Can you work these out from the model? Positions are in its coordinate system, mm. Give positions to 0.01 mm unless a question says otherwise; leave off trailing zeros. Loops run counter-clockwise (first coordinate to the right, second up) from the corner with the lowest first, then second, coordinate; pieces in that order, holes last. Notation, with made-up numbers: M -12.5,60 L 7.5,60 A24 ccw 7.5,76 Z; hole C 82,65 d4. An arc over 180 degrees is marked long. One line per item, written item: value. Start each with the question number.
from build123d import *

# Parameters (mm, degrees)
F0_W     = 5
F0_H     = 5
F1_DEPTH = 65
F2_SIZE  = 1
F3_R     = 0.65
F4_DEPTH = 6


with BuildPart() as f1:
    # F0 (on Top) → F1 (new body)
    with BuildSketch(Plane.XY):
        Rectangle(F0_W, F0_H)
    extrude(amount=F1_DEPTH)

    # F2
    f2_edges = [f1.edges().sort_by_distance(p)[0] for p in [
        (0, -2.5, 65),
        (2.5, 0, 65),
        (0, 2.5, 65),
        (-2.5, 0, 65),
    ]]
    chamfer(f2_edges, length=F2_SIZE)

    # F3 (on face) → F4 (cut)
    with BuildSketch(Plane.XY.offset(65)):
        Circle(F3_R)
    extrude(amount=-F4_DEPTH, mode=Mode.SUBTRACT)


solid = f1.part
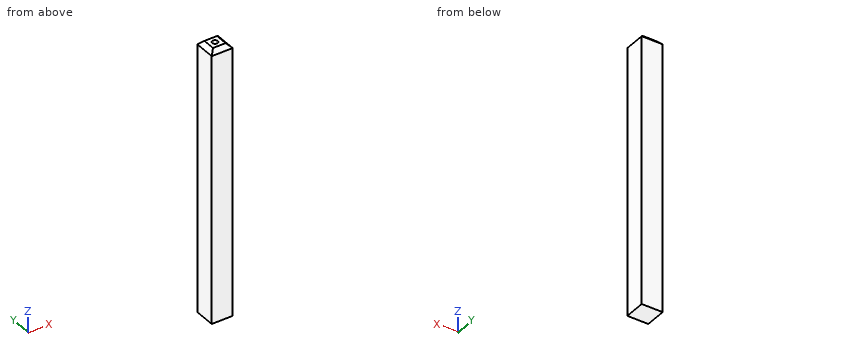
Q1. I need wall thicknesses on line 1 along Y through (x, z) = (0, 62.1); line 2 along Z through (x, y) = (-2.1, -2); line 3 along Z through (x, y) = (2.2, 0.5). Which ranges of each line are inside material? Lowest first, please.
Q2. If we section it at A-A, the plane z = 60: Write out the boundary of the cut face in (x, y).
Q3. If we section it at B-B, the plane y = 0: Write out the boundary of the cut face in (x, z).
Response:
1. line 1: -2.5 to -0.65, 0.65 to 2.5
1. line 2: 0 to 64.4
1. line 3: 0 to 64.3
2. outline: M -2.5,-2.5 L 2.5,-2.5 L 2.5,2.5 L -2.5,2.5 Z; hole C 0,0 d1.3
3. outline: M -2.5,0 L 2.5,0 L 2.5,64 L 1.5,65 L 0.65,65 L 0.65,59 L -0.65,59 L -0.65,65 L -1.5,65 L -2.5,64 Z
